Read the model definition and answer for the solid it produces. Units are mm, in the model's axes. Coordinates: 2 decimals unless noted, no trailing zeros. Loops run counter-clockwise (first coordinate to the right, second up) from the corner with the lowest first, then second, coordinate; pieces in that order, holes last.
Q1. Straight lines are drawn through the part: line 1 (Z direction, x = -28, y = 2.75); line 2 (X direction, y = 1.55, z = 13). For each, find the intervals that lie inside material, in ascending order.
Q2. Section B-B (z = 14) is taken. Give the vertices of the cut face in (x, y).
Q3. Section A-A (x = 28) is taken. Give the vertices of the cut face in (y, z).
Q4. The mould has two halves that part along Z. Classify faces 1 (the face through (0, 2, -19)), 2 (the face through (0, 2, 19)), 3 (the face through (26.712, 2.465, -14.406)), 4 (the face through (-33, 2, 0)): pulls with the +Z half, pulls with the -Z half, needs draft (parallel to the pull), parting line crosses it, or undercut.
Autodesk Inventor part; units mm, degrees
ref_plane "YZ Plane" through (0, 0, 0) normal (1, 0, 0) x (0, 1, 0)
ref_plane "XZ Plane" through (0, 0, 0) normal (0, 1, 0) x (-1, 0, 0)
ref_plane "XY Plane" through (0, 0, 0) normal (0, 0, 1) x (1, 0, 0)
sketch "Эскиз1" plane through (0, 0, 0) normal (0, 1, 0) x (-1, 0, 0)
  line L0 (33, -19) -> (-33, -19)
  line L1 (-33, -19) -> (-33, 19)
  line L2 (-33, 19) -> (33, 19)
  line L3 (33, 19) -> (33, -19)
  line L4 (0, -26.6) -> (0, 26.6)
  line L5 (46.2, 0) -> (-46.2, 0)
  circle A0 centre (28, -14) radius 1.35
  circle A1 centre (28, 14) radius 1.35
  circle A2 centre (-28, -14) radius 1.35
  circle A3 centre (-28, 14) radius 1.35
  point P0 (0, 0)
  dimension "d0" = 66
  dimension "d1" = 38
  dimension "d11" = 2.7
  dimension "d12" = 5
  dimension "d13" = 5
extrude "Выдавливание1" add sketch "Эскиз1" along normal blind 5
properties part number "драйвер двигателя"
Numbers:
1. line 1: z = -19 to -15.35, -12.65 to 12.65, 15.35 to 19
1. line 2: x = -33 to -28.91, -27.09 to 27.09, 28.91 to 33
2. outline: (-33, 0) - (-29.35, 0) - (-29.35, 5) - (-33, 5) - close; (-26.65, 0) - (26.65, 0) - (26.65, 5) - (-26.65, 5) - close; (29.35, 0) - (33, 0) - (33, 5) - (29.35, 5) - close
3. outline: (0, -19) - (5, -19) - (5, -15.35) - (0, -15.35) - close; (0, -12.65) - (5, -12.65) - (5, 12.65) - (0, 12.65) - close; (0, 15.35) - (5, 15.35) - (5, 19) - (0, 19) - close
4. face 1: pulls with the -Z half
4. face 2: pulls with the +Z half
4. face 3: undercut
4. face 4: needs draft
